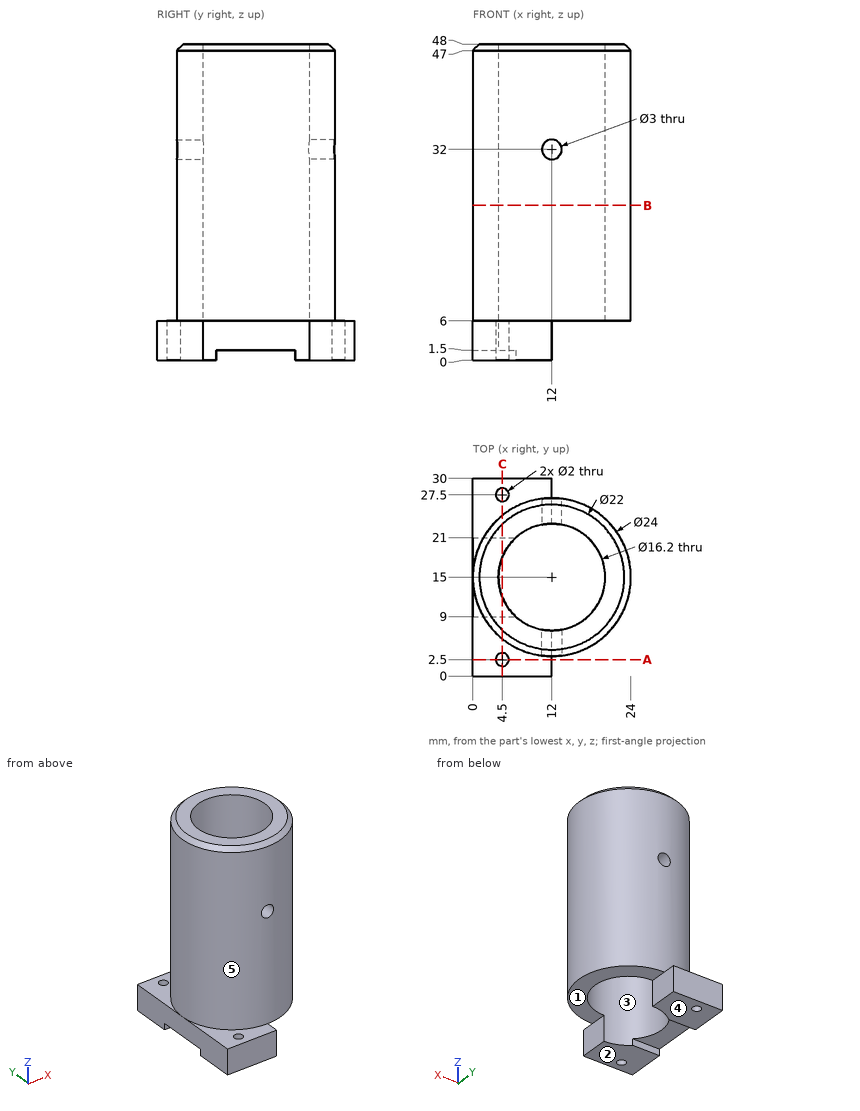
Input: dimensioned drawing with shaded views. Units: mm. Origin: part minimum x, y, z. A direction names the side the tool comes from. Give positions to 0.01 mm unless a question says otherwise; leave off trailing zeros. Order: outer loops, then holes, each group sorted by start corner. A loop starts at its lowest first (then second) coordinate and runs counter-clockwise, first axis right, second up.
(1) Material intervals for line 1 along Y through (x, z) = (12, 21.5); line 2 along Y through (x, z) = (5.5, 23.5); line 3 along X through (y, z) = (21, 4), sorted ascending.
(2) Pull-direction query (Y, two-part tool) for the marked faces 3, 4 and 5; classes: +Y half, -Y half, draft (parallel to the pull), parting line (faces both ways), or undercut.
(3) Section query A-A (y = 2.5). Return the cut outline in (x, z), plus the area to 3 significant figures.
(4) Access query for the marked faces 1 and 2. Directions: +Z, -Z, +X, -X, +Y, -Y. A direction counts if a zero-diameter tool reaches every point of the face in a straight line with its end or side. Return the directions, or none.
(5) Contact query for flat-ended pins moving along their axis: P1, Ø1.5, axis at y = 10, z = 13.5, coming from the -X side; P2, Ø2, axis at y = 12.5, z = 9, coming from the +X side; P3, Ø1.5, axis at x = 16, z = 11.5, coming from the -Y side. Output: stop coordinate, or through.
(6) Section query C-C (x = 4.5). State how many separate pieces and enclosed holes the cut face has, plus the area to 3 significant figures.
(7) Section query B-B (z = 23.5). Return the cut outline in (x, y), plus the area to 3 significant figures.
Outcome:
1. line 1: y = 3 to 6.9, 23.1 to 27
1. line 2: y = 4.91 to 10.17, 19.83 to 25.09
1. line 3: x = 0 to 6.56
2. face 3: undercut
2. face 4: draft
2. face 5: parting line
3. outline: (0, 0) - (3.5, 0) - (3.5, 6) - (0, 6) - close; (5.5, 0) - (12, 0) - (12, 6) - (5.5, 6) - close
3. area: 60.0 mm2
4. face 1: -Z, +X, +Y, -Y
4. face 2: -Z, +X, -X, +Y, -Y
5. P1: stops at x = 0.78
5. P2: stops at x = 23.91
5. P3: stops at y = 3.45
6. separate pieces: 4
6. enclosed holes: 0
6. area: 639 mm2
7. outline: circle Ø24 at (12, 15); hole circle Ø16.2 at (12, 15)
7. area: 246 mm2
